Design review of the part built by this model. Coordinates are the model's own, in mm. A direction names the side the tool comes from. Give positions to 0.01 mm unless a question says otherwise; leave off trailing zeros. Order: outer loops, then holes, each group sorted by start corner. A loop starts at its lowest first (then second) coordinate and runs counter-clockwise, first axis right, second up. Notation, with made-up numbers: (75, 1) -> (84, 1) arc R24 cw to (84, 17) -> close; hole circle Ø10 at (14, 77.25). An arc over 180 degrees is marked (long way). Return JSON: item names as keys, results as strings.
```python
from build123d import *

# Parameters (mm, degrees)
F0_W     = 3
F0_H     = 18
F0_H_2   = 19.675914
F1_DEPTH = 25
F4_D     = 6.5
F5_D     = 6.5
F6_R     = 3
F7_R     = 6


with BuildPart() as f1:
    # F0 (on Front) → F1 (new body)
    with BuildSketch(Plane.XZ):
        Polygon((110, 1.5), (-110, 1.5), (-110, -1.5), (-107, -1.5), (107, -1.5), (110, -1.5), align=None)
        with Locations((-108.5, -10.5)):
            Rectangle(F0_W, F0_H)
        with Locations((108.5, -11.337957)):
            Rectangle(F0_W, F0_H_2)
    extrude(amount=F1_DEPTH)

    # F4 (through all)
    with Locations(Plane.XY.offset(1.5)):
        with Locations((-90, -19.5), (-90, -6.5), (90, -6.5), (90, -19.5)):
            Hole(F4_D / 2)

    # F5 (through all)
    with Locations(Plane(origin=(-110, 0, 0), x_dir=(0, -1, 0), z_dir=(-1, 0, 0))):
        with Locations((19.5, -11.5), (6.5, -11.5)):
            Hole(F5_D / 2)

    # F6
    f6_edges = [f1.edges().sort_by_distance(p)[0] for p in [
        (-107, -12.5, -1.5),
        (107, -12.5, -1.5),
    ]]
    fillet(f6_edges, radius=F6_R)

    # F7
    f7_edges = [f1.edges().sort_by_distance(p)[0] for p in [
        (-110, -12.5, 1.5),
        (110, -12.5, 1.5),
    ]]
    fillet(f7_edges, radius=F7_R)


solid = f1.part
```
Item 1: Machinability: for faces 4 (the face through (107, -12, -13)), 5 (the face through (-86.753, -6.357, -0.021)), which of the approach directions +Z, -Z, +X, -X, +Y, -Y give a long, thin tool a straight path to every point of the face, cutting with its end or side? Answer none if there is none.
Result set:
{"face 4": "-Z, +Y, -Y", "face 5": "+Z, -Z"}
Item 2: Mouldability with a two-part tool opening along X and no side actions: class faces 1 (the face through (110, -12, -13)), 2 (the face through (-107, -12, -12)), 3 (the face through (-108.479, -22.747, -11.357)) as released by +X, released by -X, zero draft, split by the parting line, or undercut.
Result set:
{"face 1": "released by +X", "face 2": "undercut", "face 3": "zero draft"}
Item 3: Wall thickness on L1, parallel to Y at x = 90, z = 0.75; L2, parallel to X at y = -15, z = -14.25; L3, parallel to Z at x = 17, y = -13.75: over which ranges is each line inside the solid? List them lowest first. Write a range as [from, to].
Result set:
{"L1": "y = [-25, -22.75], [-16.25, -9.75], [-3.25, 0]", "L2": "x = [-110, -107], [107, 110]", "L3": "z = [-1.5, 1.5]"}
Item 4: Add section B-B (z = -11.5). Give the boundary of the cut face in (x, y), plus the area to 3 significant figures.
Result set:
{"outline": "(-110, -25) -> (-107, -25) -> (-107, -22.75) -> (-110, -22.75) -> close; (-110, -16.25) -> (-107, -16.25) -> (-107, -9.75) -> (-110, -9.75) -> close; (-110, -3.25) -> (-107, -3.25) -> (-107, 0) -> (-110, 0) -> close; (107, -25) -> (110, -25) -> (110, -22.75) -> (107, -22.75) -> close; (107, -16.25) -> (110, -16.25) -> (110, -9.75) -> (107, -9.75) -> close; (107, -3.25) -> (110, -3.25) -> (110, 0) -> (107, 0) -> close", "area": "72.0 mm^2"}
Item 5: Add section A-A (y = -19.5). Give the boundary of the cut face in (x, z), plus the area to 3 significant figures.
Result set:
{"outline": "(-110, -19.5) -> (-107, -19.5) -> (-107, -14.75) -> (-110, -14.75) -> close; (-110, -8.25) -> (-107, -8.25) -> (-107, -4.5) arc R3 cw to (-104, -1.5) -> (-93.25, -1.5) -> (-93.25, 1.5) -> (-104, 1.5) arc R6 ccw to (-110, -4.5) -> close; (-86.75, -1.5) -> (86.75, -1.5) -> (86.75, 1.5) -> (-86.75, 1.5) -> close; (93.25, -1.5) -> (104, -1.5) arc R3 cw to (107, -4.5) -> (107, -8.25) -> (110, -8.25) -> (110, -4.5) arc R6 ccw to (104, 1.5) -> (93.25, 1.5) -> close; (107, -21.18) -> (110, -21.18) -> (110, -14.75) -> (107, -14.75) -> close", "area": "683 mm^2"}
Item 6: Add section C-C (x = 90). Give the boundary of the cut face in (y, z).
Result set:
{"outline": "(-25, -1.5) -> (-22.75, -1.5) -> (-22.75, 1.5) -> (-25, 1.5) -> close; (-16.25, -1.5) -> (-9.75, -1.5) -> (-9.75, 1.5) -> (-16.25, 1.5) -> close; (-3.25, -1.5) -> (0, -1.5) -> (0, 1.5) -> (-3.25, 1.5) -> close"}
Item 7: For pin 1 (8 mm diameter, centred on x = -20, y = -21.5, fed in from -Z); pin 2 (6 mm diameter, centred on x = 90, y = -6.5, fed in from +Z); pin 3 (1 mm diameter, centred on y = -9.5, z = -3.5, fed in from -X); pin 4 (3.5 mm diameter, centred on x = -108, y = -12.5, fed in from -Z), all flat-tipped, find the tip position at first contact; note any pin that passes through.
Result set:
{"pin 1": "stops at z = -1.5", "pin 2": "passes through", "pin 3": "stops at x = -109.98", "pin 4": "stops at z = -19.5"}
